from build123d import *

# Parameters (mm, degrees)
F0_R          = 4.125
F0_R_2        = 1.7
F0_R_3        = 11.75
F1_DEPTH      = 6.13
F3_DEPTH      = 35
F4_R          = 4.5
F5_DEPTH      = 10
F6_R          = 4.25
F7_DEPTH      = 10
F8_R          = 7
F9_DEPTH      = 3
F10_R         = 7
F11_DEPTH     = 3
F13_R         = 5
F12_R         = 3.5
F14_DEPTH     = 2.9
F15_R         = 3.5
F16_DEPTH     = 5
F17_T1_DEPTH  = 32.5
F17_T3_DEPTH  = 9.3301270189
F17_T5_DEPTH  = 36.6690475583
F17_T7_DEPTH  = 7.5391052434
F17_T9_DEPTH  = 36.6690475583
F17_T12_ANGLE = 90
F17_T14_ANGLE = 45
F17_T16_ANGLE = 45
F17_T18_ANGLE = 90
F18_R         = 1
F19_DEPTH     = 28.87


# Not quite as in the source:
# - a fillet or chamfer that OpenCascade refuses, or shapes differently, is made with other operations: its cross-section is extruded or revolved along the edge and cut away or added


with BuildPart() as f1:
    # F0 (on Top) → F1 (new body)
    with BuildSketch(Plane.XY):
        Polygon((-29.6984848098, 0), (0, 0), (29.6984848098, 0), (29.6984848098, 29.7), (0, 59.3984848098), (-29.6984848098, 29.7), align=None)
        with Locations((-20.59, 7.3196897832)):
            Circle(F0_R, mode=Mode.SUBTRACT)
        with Locations((0, 7.7796897832)):
            Circle(F0_R_2, mode=Mode.SUBTRACT)
        with Locations((20.59, 7.3196897832)):
            Circle(F0_R, mode=Mode.SUBTRACT)
        with Locations((-21.9203102168, 29.7)):
            Circle(F0_R_2, mode=Mode.SUBTRACT)
        with Locations((0, 29.7)):
            Circle(F0_R_3, mode=Mode.SUBTRACT)
        with Locations((21.9203102168, 29.7)):
            Circle(F0_R_2, mode=Mode.SUBTRACT)
        with Locations((0, 51.6203102168)):
            Circle(F0_R_2, mode=Mode.SUBTRACT)
    extrude(amount=F1_DEPTH)

    # F2 (on face) → F3 (join)
    with BuildSketch(Plane(origin=(0, 0, 0), x_dir=(1, 0, 0), z_dir=(0, 0, -1))):
        Polygon((0, -59.3984848098), (-29.6984848098, -29.7), (-36.7695526217, -36.7710678119), (-5.8406204336, -67.7), (0, -67.7), (5.8406204336, -67.7), (36.7695526217, -36.7710678119), (29.6984848098, -29.7), align=None)
    extrude(amount=-F3_DEPTH)

    # F4 (on face) → F5 (cut, through all)
    with BuildSketch(Plane(origin=(-29.6992424049, 29.6992424049, 0), x_dir=(0.7071067812, 0.7071067812, 0), z_dir=(0.7071067812, -0.7071067812, 0))):
        with Locations((16.6010714012, 21.13)):
            Circle(F4_R)
    extrude(amount=-F5_DEPTH, mode=Mode.SUBTRACT)

    # F6 (on face) → F7 (cut, through all)
    with BuildSketch(Plane(origin=(29.6992424049, 29.6992424049, 0), x_dir=(0.7071067812, -0.7071067812, 0), z_dir=(-0.7071067812, -0.7071067812, 0))):
        with Locations((-16.6010714012, 21.13)):
            Circle(F6_R)
    extrude(amount=-F7_DEPTH, mode=Mode.SUBTRACT)

    # F8 (on face) → F9 (cut)
    with BuildSketch(Plane(origin=(-36.7703102168, 36.7703102168, 0), x_dir=(-0.7071067812, -0.7071067812, 0), z_dir=(-0.7071067812, 0.7071067812, 0))):
        with Locations((-16.6010714006, 21.13)):
            Circle(F8_R)
    extrude(amount=-F9_DEPTH, mode=Mode.SUBTRACT)

    # F10 (on face) → F11 (cut)
    with BuildSketch(Plane(origin=(36.7703102168, 36.7703102168, 0), x_dir=(-0.7071067812, 0.7071067812, 0), z_dir=(0.7071067812, 0.7071067812, 0))):
        with Locations((16.6010714007, 21.13)):
            Circle(F10_R)
    extrude(amount=-F11_DEPTH, mode=Mode.SUBTRACT)

    # F13
    f13_edges = [f1.edges().sort_by_distance(p)[0] for p in [
        (33.234019, 33.235534, 35),
        (-33.234019, 33.235534, 35),
        (29.698485, 29.7, 3.065),
        (29.698485, 0, 3.065),
        (-29.698485, 0, 3.065),
        (-29.698485, 29.7, 3.065),
        (-5.84062, 67.7, 17.5),
        (5.84062, 67.7, 17.5),
    ]]
    fillet(f13_edges, radius=F13_R)

    # F12 (on face) → F14 (cut)
    with BuildSketch(Plane.XY.offset(6.13)):
        with Locations((0, 51.6203102168)):
            Circle(F12_R)
        with Locations((-21.9203102168, 29.7)):
            Circle(F12_R)
        with Locations((21.9203102168, 29.7)):
            Circle(F12_R)
        with Locations((0, 7.7796897832)):
            Circle(F12_R)
    extrude(amount=-F14_DEPTH, mode=Mode.SUBTRACT)

    # F15 (on face) → F16 (join)
    with BuildSketch(Plane.XY.offset(6.13)):
        Polygon((16.692885683, 14.0696897832), (-16.692885683, 14.0696897832), (-12.7957713659, 7.3196897832), (-16.692885683, 0.5696897832), (16.692885683, 0.5696897832), (12.7957713659, 7.3196897832), align=None)
        with Locations((0, 7.7796897832)):
            Circle(F15_R, mode=Mode.SUBTRACT)
        Polygon((16.692885683, 0.5696897832), (-16.692885683, 0.5696897832), (-17.0217962327, 0), (0, 0), (17.0217962327, 0), align=None)
        Polygon((-17.0217962327, 14.6393795664), (-16.692885683, 14.0696897832), (16.692885683, 14.0696897832), (17.0217962327, 14.6393795664), (0, 14.6393795664), align=None)
    extrude(amount=F16_DEPTH)

    # F17: fillet of radius 1 on 13 edges, made by hand

    # F17_s2 → F17_t1 (cut)
    with BuildSketch(Plane.XY.offset(-2.5)):
        with BuildLine():
            ThreePointArc((36.0624458405, 37.4781745931), (36.3553390593, 36.7710678119), (36.0624458405, 36.0639610307))
            Line((36.0624458405, 36.0639610307), (36.7695526217, 36.7710678119))
            Line((36.7695526217, 36.7710678119), (36.0624458405, 37.4781745931))
        make_face()
        with BuildLine():
            ThreePointArc((-36.0624458405, 36.0639610307), (-36.3553390593, 36.7710678119), (-36.0624458405, 37.4781745931))
            Line((-36.0624458405, 37.4781745931), (-36.7695526217, 36.7710678119))
            Line((-36.7695526217, 36.7710678119), (-36.0624458405, 36.0639610307))
        make_face()
    extrude(amount=F17_T1_DEPTH, mode=Mode.SUBTRACT)

    # F17_s4 → F17_t3 (cut)
    with BuildSketch(Plane.XY.offset(6.13)):
        with BuildLine():
            ThreePointArc((-15.2897454251, 0), (-16.1557708289, 0.5), (-16.1557708289, 1.5))
            Line((-16.1557708289, 1.5), (-17.0217962327, 0))
            Line((-17.0217962327, 0), (-15.2897454251, 0))
        make_face()
        with BuildLine():
            ThreePointArc((-15.2897454251, 14.6393795664), (-16.1557708289, 14.1393795664), (-16.1557708289, 13.1393795664))
            Line((-16.1557708289, 13.1393795664), (-17.0217962327, 14.6393795664))
            Line((-17.0217962327, 14.6393795664), (-15.2897454251, 14.6393795664))
        make_face()
        with BuildLine():
            ThreePointArc((16.1557708289, 13.1393795664), (16.1557708289, 14.1393795664), (15.2897454251, 14.6393795664))
            Line((15.2897454251, 14.6393795664), (17.0217962327, 14.6393795664))
            Line((17.0217962327, 14.6393795664), (16.1557708289, 13.1393795664))
        make_face()
        with BuildLine():
            ThreePointArc((15.2897454251, 0), (16.1557708289, 0.5), (16.1557708289, 1.5))
            Line((16.1557708289, 1.5), (17.0217962327, 0))
            Line((17.0217962327, 0), (15.2897454251, 0))
        make_face()
    extrude(amount=F17_T3_DEPTH, mode=Mode.SUBTRACT)

    # F17_s6 → F17_t5 (cut)
    with BuildSketch(Plane(origin=(3.536291501, 3.536291501, 0), x_dir=(0, 0, 1), z_dir=(0.7071067812, 0.7071067812, 0))):
        with BuildLine():
            ThreePointArc((34, -52.0010714012), (34.7071067812, -51.7081781824), (35, -51.0010714012))
            Line((35, -51.0010714012), (35, -52.0010714012))
            Line((35, -52.0010714012), (34, -52.0010714012))
        make_face()
    extrude(amount=F17_T5_DEPTH, mode=Mode.SUBTRACT)

    # F17_s8 → F17_t7 (cut)
    with BuildSketch(Plane.YZ.offset(-3.7695526217)):
        with BuildLine():
            ThreePointArc((67.7, 34), (67.4071067812, 34.7071067812), (66.7, 35))
            Line((66.7, 35), (67.7, 35))
            Line((67.7, 35), (67.7, 34))
        make_face()
    extrude(amount=F17_T7_DEPTH, mode=Mode.SUBTRACT)

    # F17_s10 → F17_t9 (cut)
    with BuildSketch(Plane(origin=(-29.4652236891, 29.4652236891, 0), x_dir=(0, 0, 1), z_dir=(0.7071067812, -0.7071067812, 0))):
        with BuildLine():
            ThreePointArc((34, -52.0010714012), (34.7071067812, -51.7081781824), (35, -51.0010714012))
            Line((35, -51.0010714012), (35, -52.0010714012))
            Line((35, -52.0010714012), (34, -52.0010714012))
        make_face()
    extrude(amount=F17_T9_DEPTH, mode=Mode.SUBTRACT)

    # F17_s11 → F17_t12 (revolve, cut)
    with BuildSketch(Plane.XY.offset(30)):
        with BuildLine():
            ThreePointArc((-36.0624458405, 37.4781745931), (-36.3553390593, 36.7710678119), (-36.0624458405, 36.0639610307))
            Line((-36.0624458405, 36.0639610307), (-36.7695526217, 36.7710678119))
            Line((-36.7695526217, 36.7710678119), (-36.0624458405, 37.4781745931))
        make_face()
    revolve(axis=Axis((-33.2340187158, 40.3066017178, 30), (-0.7071067812, 0.7071067812, 0)), revolution_arc=F17_T12_ANGLE, mode=Mode.SUBTRACT)

    # F17_s13 → F17_t14 (revolve, cut)
    with BuildSketch(Plane.YZ.offset(-3.7695526217)):
        with BuildLine():
            ThreePointArc((67.7, 34), (67.4071067812, 34.7071067812), (66.7, 35))
            Line((66.7, 35), (67.7, 35))
            Line((67.7, 35), (67.7, 34))
        make_face()
    revolve(axis=Axis((-3.7695526217, 62.7, 35), (0, 0, 1)), revolution_arc=F17_T14_ANGLE, mode=Mode.SUBTRACT)

    # F17_s15 → F17_t16 (revolve, cut)
    with BuildSketch(Plane(origin=(-29.4652236891, 29.4652236891, 0), x_dir=(0, 0, 1), z_dir=(0.7071067812, -0.7071067812, 0))):
        with BuildLine():
            ThreePointArc((34, -52.0010714012), (34.7071067812, -51.7081781824), (35, -51.0010714012))
            Line((35, -51.0010714012), (35, -52.0010714012))
            Line((35, -52.0010714012), (34, -52.0010714012))
        make_face()
    revolve(axis=Axis((3.7695526217, 62.7, 35), (0, 0, 1)), revolution_arc=F17_T16_ANGLE, mode=Mode.SUBTRACT)

    # F17_s17 → F17_t18 (revolve, cut)
    with BuildSketch(Plane.XY.offset(30)):
        with BuildLine():
            ThreePointArc((36.0624458405, 37.4781745931), (36.3553390593, 36.7710678119), (36.0624458405, 36.0639610307))
            Line((36.0624458405, 36.0639610307), (36.7695526217, 36.7710678119))
            Line((36.7695526217, 36.7710678119), (36.0624458405, 37.4781745931))
        make_face()
    revolve(axis=Axis((33.2340187158, 40.3066017178, 30), (-0.7071067812, -0.7071067812, 0)), revolution_arc=F17_T18_ANGLE, mode=Mode.SUBTRACT)

    # F18 (on face) → F19 (cut, through all)
    with BuildSketch(Plane.XY.offset(35)):
        with Locations((0, 59.3984848098)):
            Circle(F18_R)
    extrude(amount=-F19_DEPTH, mode=Mode.SUBTRACT)


solid = f1.part
Can you work these out from the model? Positions are in its coordinate system, mm. A direction names the side the tool comes from. Round coordinates to 2 decimals unless told otherwise and drop trailing zeros. Write each loop counter-clockwise with the first axis right and the second up, starting at its lowest first coordinate (ties: lowest second). Pieces come first, ordered by that corner, then holes. Notation, with made-up numbers: (-35.5, 76) - (-12.5, 76) arc R15 cw to (-12.5, 105) - close; hole circle Ø6 at (48.25, 87.25). An arc over 180 degrees is marked (long way). Write each question's results on one line, items separated by ' | '. Start each with the question number.
1) Suppose I cut it at D-D (z = 18.5). List the corners of the cut face in (x, y) for me.
2) Suppose I cut it at A-A (z = 23). List the corners of the cut face in (x, y) for me, and give its area (3 significant figures).
3) Suppose I cut it at B-B (y = 19.5). List the corners of the cut face in (x, z) for me, and give its area (3 significant figures).
4) Please list where these lines run through material, in increasing order: line 1 (Y direction, x = 0, z = 2); line 2 (Y direction, x = 20.59, z = 4); line 3 (X direction, y = 5.5, z = 5).
5) For pin 1 Ø1 at (x, y) = (-20.5, 28.5) entering from -Z; pin 2 Ø2 at (y, z) = (56.5, 17.5) entering from +X; pin 3 Ø2.5 at (x, y) = (21.92, 29.7) entering from +Z; pin 4 Ø4 at (x, y) = (0, 51.62) entering from +Z, each with a flat end and sliding along its axis, tell me the tip position at first contact or that it passes through.
6) Which directions (+Z, -Z, +X, -X, +Y, -Y) give clear straight access to the entire face, cutting with the end or side of a thin tool? Please do faces 5 (the flat face through (29.698, 16, 3)), 6 (the flat face through (-33, 33, 15)), 7 (the cylindrical face through (-23.17, 30.85, 1.59)), 8 (the cylindrical face through (-20.25, 52.89, 34.7)), 9 (the flat face through (14.452, 10.189, 8.595)).
7) We'd pull the mould along Y, two halves only. Please class faces 1 (the flat face through (-29.698, 16, 3)), 2 (the flat face through (0, 67.7, 17)), 3 (the cylindrical face through (-20.305, 26.595, 4.7)), 4 (the flat face through (-23, 28, 3.23)): released by +Y, released by -Y, zero draft, split by the parting line, or undercut.
8) Suppose I cut it at C-C (z = 12.5). List the corners of the cut face in (x, y) for me, and give its area (3 significant figures).
Here are the results:
1) outline: (-36.06, 36.06) - (-29.7, 29.7) - (-20.54, 38.86) - (-25.49, 43.81) - (-27.5, 41.8) - (-29.62, 43.92) - (-36.06, 37.48) arc R1 ccw to start; (-20.44, 53.1) - (-18.32, 50.97) - (-20.33, 48.97) - (-15.38, 44.02) - (-0.71, 58.69) arc R1 cw (long way) to (0.71, 58.69) - (15.6, 43.8) - (20.55, 48.75) - (18.32, 50.97) - (20.44, 53.1) - (7.31, 66.24) arc R5 ccw to (3.77, 67.7) - (-3.77, 67.7) arc R5 ccw to (-7.31, 66.24) - close; (20.32, 39.08) - (29.7, 29.7) - (36.06, 36.06) arc R1 ccw to (36.06, 37.48) - (29.62, 43.92) - (27.5, 41.8) - (25.27, 44.03) - close
2) outline: (-36.06, 36.06) - (-29.7, 29.7) - (-20.85, 38.54) - (-25.8, 43.49) - (-27.68, 41.62) - (-29.8, 43.74) - (-36.06, 37.48) arc R1 ccw to start; (-20.26, 53.28) - (-18.14, 51.16) - (-20.02, 49.28) - (-15.07, 44.33) - (-0.71, 58.69) arc R1 cw (long way) to (0.71, 58.69) - (15.26, 44.14) - (20.21, 49.09) - (18.14, 51.16) - (20.26, 53.28) - (7.31, 66.24) arc R5 ccw to (3.77, 67.7) - (-3.77, 67.7) arc R5 ccw to (-7.31, 66.24) - close; (20.66, 38.74) - (29.7, 29.7) - (36.06, 36.06) arc R1 ccw to (36.06, 37.48) - (29.8, 43.74) - (27.68, 41.62) - (25.61, 43.69) - close | area: 710 mm2
3) outline: (-29.7, 0) - (-5.83, 0) - (-5.83, 6.13) - (-29.7, 6.13) - close; (5.83, 0) - (29.7, 0) - (29.7, 6.13) - (5.83, 6.13) - close | area: 293 mm2
4) line 1: y = 0 to 6.08, 9.48 to 17.95, 41.45 to 49.92, 53.32 to 67.7 | line 2: y = 0 to 3.19, 11.44 to 26.46, 32.94 to 52.95 | line 3: x = -29.7 to -24.29, -16.89 to -2.66, 2.66 to 16.89, 24.29 to 29.7
5) pin 1: stops at z = 0 | pin 2: stops at x = 18.04 | pin 3: passes through | pin 4: stops at z = 3.23
6) face 5: +Z, -Z, +X, -Y | face 6: +Z, -X, -Y | face 7: +Z, -Z | face 8: +Z, -X, +Y | face 9: +Z, +X
7) face 1: zero draft | face 2: released by +Y | face 3: undercut | face 4: undercut
8) outline: (-36.06, 36.06) - (-29.7, 29.7) - (-0.71, 58.69) arc R1 cw (long way) to (0.71, 58.69) - (29.7, 29.7) - (36.06, 36.06) arc R1 ccw to (36.06, 37.48) - (7.31, 66.24) arc R5 ccw to (3.77, 67.7) - (-3.77, 67.7) arc R5 ccw to (-7.31, 66.24) - (-36.06, 37.48) arc R1 ccw to start | area: 902 mm2
